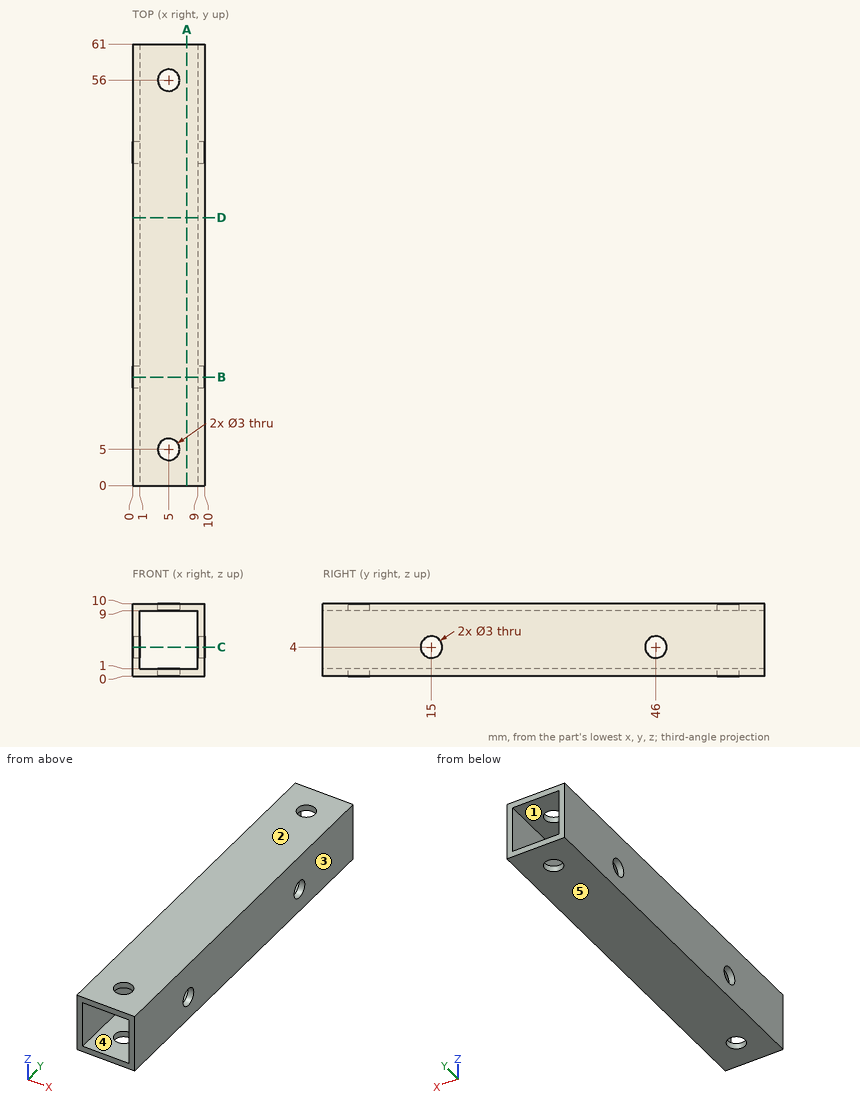
Here's the drawing with two shaded views (mm, measured from the low corner). I have some questions. A direction names the side the tool comes from. Coordinates: 2 decimals unless noted, no trailing zeros. Order: outer loops, then holes, each group sorted by start corner. A loop starts at its lowest first (then second) coordinate and runs counter-clockwise, first axis right, second up. Notation, with made-up numbers: (-27.75, 72.25) - (20.25, 72.25) arc R10 ccw to (20.25, 85.25) - close; hole circle Ø2 at (36, 75). An arc over 180 degrees is marked (long way). Answer in a Markdown table with one row per item. Add a question column.
(1) If we section it at C-C, the plane z = 4: Please give me the cut outline in (x, y), then the cut area to 3 significant figures.
(2) Will this pin go through, and if not, where does the flat tip stop? pin 1 (1 mm diameter, centred on y = 12.5, z = 5.5, fed in from -X).
(3) If we section it at A-A, the plane x = 7.5: Please give me the cut outline in (y, z), then the cut area to 3 significant figures.
(4) If we section it at D-D, the plane y = 37: Please give me the cut outline in (x, z), then the cut area to 3 significant figures.
(5) On a 3-axis mill with a long thin cutter (end or side, diameter ignored), from which of +Z, -Z, +X, -X, +Y, -Y can I reach the whole of each face in a straight line? I mean the marked faces 1 and 2. Say none if no direction works.
(6) If we mould it in two halves opening along X, with no side actions, what happens to the marked faces 3, 4 and 5? For each: released by +X, released by -X, zero draft, split by the parting line, or undercut.
(7) If we section it at B-B, the plane y = 15: Please give me the cut outline in (x, z), then the cut area to 3 significant figures.
(8) I need wall thicknesses on L1, parallel to Y at x = 5, z = 0.5; L2, parallel to X at y = 12, z = 6.5. Which ranges of each line are inside material? Lowest first, please.
Results are:
| question | item | result |
|---|---|---|
| 1 | outline | (0, 0) - (1, 0) - (1, 13.5) - (0, 13.5) - close; (0, 16.5) - (1, 16.5) - (1, 44.5) - (0, 44.5) - close; (0, 47.5) - (1, 47.5) - (1, 61) - (0, 61) - close; (9, 0) - (10, 0) - (10, 13.5) - (9, 13.5) - close; (9, 16.5) - (10, 16.5) - (10, 44.5) - (9, 44.5) - close; (9, 47.5) - (10, 47.5) - (10, 61) - (9, 61) - close |
| 1 | area | 110 mm2 |
| 2 | pin 1 | stops at x = 0 |
| 3 | outline | (0, 0) - (61, 0) - (61, 1) - (0, 1) - close; (0, 9) - (61, 9) - (61, 10) - (0, 10) - close |
| 3 | area | 122 mm2 |
| 4 | outline | (0, 0) - (10, 0) - (10, 10) - (0, 10) - close; hole (1, 1) - (9, 1) - (9, 9) - (1, 9) - close |
| 4 | area | 36.0 mm2 |
| 5 | face 1 | +Y, -Y |
| 5 | face 2 | +Z, +X, -X, +Y, -Y |
| 6 | face 3 | released by +X |
| 6 | face 4 | undercut |
| 6 | face 5 | zero draft |
| 7 | outline | (0, 0) - (10, 0) - (10, 2.5) - (9, 2.5) - (9, 1) - (1, 1) - (1, 2.5) - (0, 2.5) - close; (0, 5.5) - (1, 5.5) - (1, 9) - (9, 9) - (9, 5.5) - (10, 5.5) - (10, 10) - (0, 10) - close |
| 7 | area | 30.0 mm2 |
| 8 | L1 | y = 0 to 3.5, 6.5 to 54.5, 57.5 to 61 |
| 8 | L2 | x = 0 to 1, 9 to 10 |
